```python
from build123d import *

# Parameters (mm, degrees)
SKETCH2_R          = 3.75
CUT_EXTRUDE1_DEPTH = 15
SKETCH3_R          = 1.5
CUT_EXTRUDE2_DEPTH = 10
FILLET1_R          = 0.5


with BuildPart() as part:
    # Sketch1 → Revolve1 (revolve)
    with BuildSketch(Plane(origin=(0, 0, 0), x_dir=(1, 0, 0), z_dir=(0, 1, 0))):
        Polygon((0, 0), (0, 7.5), (22, 7.5), (22, 2.5), (49.2, 2.5), (49.2, 0), align=None)
    revolve(axis=Axis((49.2, 0, 0), (-1, 0, 0)))

    # Sketch2 → Cut-Extrude1 (cut)
    with BuildSketch(Plane.ZY):
        Circle(SKETCH2_R)
    extrude(amount=-CUT_EXTRUDE1_DEPTH, mode=Mode.SUBTRACT)

    # Sketch3 → Cut-Extrude2 (cut)
    with BuildSketch(Plane.XY):
        with Locations((4.905983841, 0)):
            Circle(SKETCH3_R)
    extrude(amount=-CUT_EXTRUDE2_DEPTH, mode=Mode.SUBTRACT)

    # Fillet1
    fillet1_edges = [part.edges().sort_by_distance(p)[0] for p in [
        (4.905983841, 1.5, -7.348469228),
    ]]
    fillet(fillet1_edges, radius=FILLET1_R)


solid = part.part
```
Part model, mm, in its own coordinate system. A direction names the side the tool comes from. Coordinates: 2 decimals unless noted, no trailing zeros. Order: outer loops, then holes, each group sorted by start corner. A loop starts at its lowest first (then second) coordinate and runs counter-clockwise, first axis right, second up. Notation, with made-up numbers: (19, 81) - (47, 81) arc R22 cw to (47, 97) - close; hole circle Ø9 at (45.25, 45). An arc over 180 degrees is marked (long way). Return JSON: item names as keys, results as strings. Group by question number.
Item 1: Which spindle directions (+Z, -Z, +X, -X, +Y, -Y) get a long thin tool onto all of the face, cutting with end or side? Do faces 1 (the face through (11.154, -2.253, -7.154)), 2 (the face through (7.395, 1.126, 3.577)). Say none if no direction does.
Item 2: Cut at D-D (x = 30). List the corners of the cut face in (y, z).
Item 3: Cut at C-C (y = 5.25). List the corners of the cut face in (x, z).
Item 4: Pull direction X, two halves, no side cores. Call faces 3 (the face through (35.79, 2.44, 0.54)), 4 (the face through (0, 3, 3)), 5 (the face through (22, -2, 2)), 6 (the face through (5.712, 1.265, -5.194)): pulls with the +X half, pulls with the -X half, needs draft (parallel to the pull), parting line crosses it, or undercut.
Item 5: Drill centre lines: probe 1 along X at (y, z) = (0, -5.15); probe 2 along X at (y, z) = (2.25, -4.25); probe 3 along X at (y, z) = (-2.75, -1.5). Where is each one in solid material? Low to high. Write a range as from..to.
Item 6: Cut at B-B (x = 16.5). List the corners of the cut face in (y, z), plus the area to 3 significant figures.
Item 7: Cut at A-A (z = 0). List the corners of the cut face in (x, y).
Item 8: Pin check, flat tips, straight feed: pin 1 (4 mm diameter, centred on x = 16, y = 3.5, fed in from -Z); pin 2 (4 mm diameter, centred on y = 2.5, z = -4.5, fed in from +X); pin 3 (1 mm diameter, centred on x = 18.5, z = 2.5, fed in from +Y). Stop position of each tip, or through.
Check values:
{
 "1": {"face 1": "+X, -X", "face 2": "-X"},
 "2": {"outline": "circle Ø5 at (0, 0)"},
 "3": {"outline": "(0, -5.36) - (22, -5.36) - (22, 5.36) - (0, 5.36) - close"},
 "4": {"face 3": "needs draft", "face 4": "pulls with the -X half", "face 5": "pulls with the +X half", "face 6": "undercut"},
 "5": {"probe 1": "x = 0..3.41, 6.41..22", "probe 2": "x = 0..22", "probe 3": "x = 15..22"},
 "6": {"outline": "circle Ø15 at (0, 0)", "area": "177 mm2"},
 "7": {"outline": "(0, -7.5) - (22, -7.5) - (22, -2.5) - (49.2, -2.5) - (49.2, 2.5) - (22, 2.5) - (22, 7.5) - (0, 7.5) - (0, 3.75) - (15, 3.75) - (15, -3.75) - (0, -3.75) - close"},
 "8": {"pin 1": "stops at z = -7.35", "pin 2": "stops at x = 22", "pin 3": "stops at y = 7.23"}
}
